Could you check a few things on this model? Use its own coordinates, in mm. A direction names the side the tool comes from. Coordinates: 2 decimals unless noted, no trailing zeros. Write each loop counter-clockwise with the first axis right and the second up, starting at its lowest first coordinate (ties: lowest second). Pieces come first, ordered by that corner, then holes. Notation, with made-up numbers: M 37,17 L 59,17 A33 cw 59,49 Z; hole C 64.25,-14.5 d1. An arc over 180 degrees is marked long. Answer as CSV lines item,"result". Start each with the question number.
Item 1: Suppose I cut it at A-A, the plane z = -3.5. Write out the boundary of the cut face in (x, y).
Item 2: If I drill on line 1 along Z through (x, y) = (-22, 6); line 2 along Z through (x, y) = (-93.25, 1.9), over which ranges is the centre line in solid material (lowest first)? Write a range as [from, to].
Item 3: I'm going to push flat-ended pins straight in: P1, Ø1.8, axis at x = -93.25, z = 93.25, coming from the +Y side; P2, Ø3, axis at y = 9, z = 18.75, coming from the +X side; P3, Ø5, axis at y = 10.5, z = -16, coming from the -X side; P4, Ø7, axis at x = 16.5, z = -17, coming from the +Y side. Where does each tip first touch, or does it pass through?
Item 4: On a 3-axis mill with a long thin cutter (end or side, diameter ignored), from which of +Z, -Z, +X, -X, +Y, -Y can I reach the whole of each face in a straight line? I mean faces 1 (the flat face through (-27.5, 9, 21)), 2 (the flat face through (-20.5, 9.1, -11.5)), 3 (the flat face through (-17, 9, 27.5)), 4 (the flat face through (10, 9, 21)). Say none if no direction works.
Item 5: We'd pull the mould along X, two halves only. Please class faces 5 (the flat face through (-11.5, 9, 17)), 6 (the flat face through (27.5, 9, 21)), 7 (the flat face through (-1, 0, -1)), 8 (the flat face through (10, 9, -21)): +X half, -X half, draft (parallel to the pull), parting line (faces both ways), or undercut.
```python
from build123d import *

# Parameters (mm, degrees)
SKETCH1_W                   = 195
SKETCH1_H                   = 195
BOSS_EXTRUDE1_DEPTH         = 4
SKETCH2_W                   = 17.5
SKETCH2_H                   = 17.5
BOSS_EXTRUDE2_DEPTH         = 10
SKETCH3_W                   = 14.5
SKETCH3_H                   = 14.5
CUT_EXTRUDE1_DEPTH          = 10
TAP_DRILL_FOR_M3X0_5_TAP1_D = 2.5
TAP_DRILL_FOR_M3X0_5_TAP2_D = 2.5
MIRROR2_COPY_1_SKETCH_W     = 17.5
MIRROR2_COPY_1_SKETCH_H     = 17.5
MIRROR2_COPY_1_DEPTH        = 10
MIRROR2_COPY_2_SKETCH_W     = 14.5
MIRROR2_COPY_2_SKETCH_H     = 14.5
MIRROR2_COPY_2_DEPTH        = 10
MIRROR2_COPY_3_D            = 2.5
MIRROR2_COPY_4_D            = 2.5
SKETCH8_R                   = 1.5
CUT_EXTRUDE2_DEPTH          = 4
MIRROR4_COPY_1_SKETCH_R     = 1.5
MIRROR4_COPY_1_DEPTH        = 4


with BuildPart() as part:
    # Sketch1 → Boss-Extrude1 (new body)
    with BuildSketch(Plane(origin=(0, 0, 0), x_dir=(1, 0, 0), z_dir=(0, 1, 0))):
        Rectangle(SKETCH1_W, SKETCH1_H)
    extrude(amount=BOSS_EXTRUDE1_DEPTH)

    # Sketch2 → Boss-Extrude2 (add)
    with BuildSketch(Plane(origin=(0, 4, 0), x_dir=(1, 0, 0), z_dir=(0, 1, 0))):
        with Locations((-18.75, 18.75)):
            Rectangle(SKETCH2_W, SKETCH2_H)
    boss_extrude2 = extrude(amount=BOSS_EXTRUDE2_DEPTH)

    # Sketch3 → Cut-Extrude1 (cut)
    with BuildSketch(Plane(origin=(0, 14, 0), x_dir=(1, 0, 0), z_dir=(0, 1, 0))):
        with Locations((-18.75, 18.75)):
            Rectangle(SKETCH3_W, SKETCH3_H)
    cut_extrude1 = extrude(amount=-CUT_EXTRUDE1_DEPTH, mode=Mode.SUBTRACT)

    # Tap Drill for M3x0.5 Tap1 (through all)
    with Locations(Plane.XY.offset(-10)):
        with Locations((-18.75, 9)):
            tap_drill_for_m3x0_5_tap1 = Hole(TAP_DRILL_FOR_M3X0_5_TAP1_D / 2)

    # Tap Drill for M3x0.5 Tap2 (through all)
    with Locations(Plane.ZY.offset(27.5)):
        with Locations((-18.75, 9)):
            tap_drill_for_m3x0_5_tap2 = Hole(TAP_DRILL_FOR_M3X0_5_TAP2_D / 2)

    # Mirror1: Boss-Extrude2, Cut-Extrude1, Tap Drill for M3x0.5 Tap1, Tap Drill for M3x0.5 Tap2 across plane
    add(boss_extrude2.mirror(Plane(origin=(0, 0, 0), x_dir=(1, 0, 0), z_dir=(0, 0, -1))))
    add(cut_extrude1.mirror(Plane(origin=(0, 0, 0), x_dir=(1, 0, 0), z_dir=(0, 0, -1))), mode=Mode.SUBTRACT)
    add(tap_drill_for_m3x0_5_tap1.mirror(Plane(origin=(0, 0, 0), x_dir=(1, 0, 0), z_dir=(0, 0, -1))), mode=Mode.SUBTRACT)
    add(tap_drill_for_m3x0_5_tap2.mirror(Plane(origin=(0, 0, 0), x_dir=(1, 0, 0), z_dir=(0, 0, -1))), mode=Mode.SUBTRACT)

    # Mirror2: Boss-Extrude2, Cut-Extrude1, Tap Drill for M3x0.5 Tap1, Tap Drill for M3x0.5 Tap2 across plane
    add(boss_extrude2.mirror(Plane.ZY))
    add(cut_extrude1.mirror(Plane.ZY), mode=Mode.SUBTRACT)
    add(tap_drill_for_m3x0_5_tap1.mirror(Plane.ZY), mode=Mode.SUBTRACT)
    add(tap_drill_for_m3x0_5_tap2.mirror(Plane.ZY), mode=Mode.SUBTRACT)

    # Mirror2 copy 1 sketch → Mirror2 copy 1 (add)
    with BuildSketch(Plane(origin=(0, 4, 0), x_dir=(-1, 0, 0), z_dir=(0, 1, 0))):
        with Locations((-18.75, 18.75)):
            Rectangle(MIRROR2_COPY_1_SKETCH_W, MIRROR2_COPY_1_SKETCH_H)
    extrude(amount=MIRROR2_COPY_1_DEPTH)

    # Mirror2 copy 2 sketch → Mirror2 copy 2 (cut)
    with BuildSketch(Plane(origin=(0, 14, 0), x_dir=(-1, 0, 0), z_dir=(0, 1, 0))):
        with Locations((-18.75, 18.75)):
            Rectangle(MIRROR2_COPY_2_SKETCH_W, MIRROR2_COPY_2_SKETCH_H)
    extrude(amount=-MIRROR2_COPY_2_DEPTH, mode=Mode.SUBTRACT)

    # Mirror2 copy 3 (through all)
    with Locations(Plane(origin=(0, 0, 10), x_dir=(-1, 0, 0), z_dir=(0, 0, -1))):
        with Locations((-18.75, 9)):
            Hole(MIRROR2_COPY_3_D / 2)

    # Mirror2 copy 4 (through all)
    with Locations(Plane(origin=(27.5, 0, 0), x_dir=(0, 0, -1), z_dir=(1, 0, 0))):
        with Locations((-18.75, 9)):
            Hole(MIRROR2_COPY_4_D / 2)

    # Sketch8 → Cut-Extrude2 (cut)
    with BuildSketch(Plane(origin=(0, 4, 0), x_dir=(1, 0, 0), z_dir=(0, 1, 0))):
        with Locations(Location((77.25, 93.25, 0), (0, 0, 270))):  # turned: the seam where the file's is
            Circle(SKETCH8_R)
        with Locations(Location((93.25, 93.25, 0), (0, 0, 270))):  # turned: the seam where the file's is
            Circle(SKETCH8_R)
    cut_extrude2 = extrude(amount=-CUT_EXTRUDE2_DEPTH, mode=Mode.SUBTRACT)

    # Mirror3: Cut-Extrude2 across plane
    add(cut_extrude2.mirror(Plane.ZY), mode=Mode.SUBTRACT)

    # Mirror4: Cut-Extrude2 across plane
    add(cut_extrude2.mirror(Plane(origin=(0, 0, 0), x_dir=(1, 0, 0), z_dir=(0, 0, -1))), mode=Mode.SUBTRACT)

    # Mirror4 copy 1 sketch → Mirror4 copy 1 (cut)
    with BuildSketch(Plane(origin=(0, 4, 0), x_dir=(-1, 0, 0), z_dir=(0, 1, 0))):
        with Locations(Location((77.25, 93.25, 0), (0, 0, 270))):  # turned: the seam where the file's is
            Circle(MIRROR4_COPY_1_SKETCH_R)
        with Locations(Location((93.25, 93.25, 0), (0, 0, 270))):  # turned: the seam where the file's is
            Circle(MIRROR4_COPY_1_SKETCH_R)
    extrude(amount=-MIRROR4_COPY_1_DEPTH, mode=Mode.SUBTRACT)


solid = part.part
```
Ans:
1,outline,"M -97.5,0 L 97.5,0 L 97.5,4 L -97.5,4 Z"
2,line 1,"z = [-27.5, -26], [-11.5, -10], [10, 11.5], [26, 27.5]"
2,line 2,"z = [-97.5, -94.75], [-91.75, 91.75], [94.75, 97.5]"
3,P1,"passes through"
3,P2,"stops at x = 27.5"
3,P3,"stops at x = -27.5"
3,P4,"stops at y = 4"
4,face 1,"+Z, -Z, -X, +Y"
4,face 2,"+Y"
4,face 3,"+Z, +X, -X, +Y"
4,face 4,"+Z, -Z, +Y"
5,face 5,"undercut"
5,face 6,"+X half"
5,face 7,"draft"
5,face 8,"undercut"
